Geometry: final body of the model. Coordinates: model frame, mm. A direction names the side the tool comes from. Coordinates: 2 decimals unless noted, no trailing zeros. Loops run counter-clockwise (first coordinate to the right, second up) from the corner with the lowest first, then second, coordinate; pieces in that order, holes last. Notation, with made-up numbers: (-18.75, -11) - (22.25, -11) arc R32 cw to (22.25, 21) - close; hole circle Ø10 at (27, 66.25). An arc over 180 degrees is marked (long way). Answer in a Markdown table with one row per item.
from build123d import *

# Parameters (mm, degrees)
SKETCH1_W           = 101.6
SKETCH1_H           = 101.6
BOSS_EXTRUDE1_DEPTH = 101.6
SKETCH3_W           = 50.8
SKETCH3_H           = 101.6
REVOLVE1_ANGLE      = 90
FILLET1_R           = 2.54


with BuildPart() as part:
    # Sketch1 → Boss-Extrude1 (new body)
    with BuildSketch(Plane(origin=(0, 0, 0), x_dir=(1, 0, 0), z_dir=(0, 1, 0))):
        Rectangle(SKETCH1_W, SKETCH1_H)
    extrude(amount=BOSS_EXTRUDE1_DEPTH)

    # Sketch3 → Revolve1 (revolve)
    with BuildSketch(Plane.XY.offset(50.8)):
        with Locations((25.4, 50.8)):
            Rectangle(SKETCH3_W, SKETCH3_H)
    revolve(axis=Axis((0, 0, 50.8), (0, -1, 0)), revolution_arc=REVOLVE1_ANGLE)

    # Fillet1
    fillet1_edges = [part.edges().sort_by_distance(p)[0] for p in [
        (0, 50.8, 50.8),
    ]]
    fillet(fillet1_edges, radius=FILLET1_R)


solid = part.part
(1) Cut plane B-B on x = -17. Output: boundary loops of the cut face in (y, z).
Verdict:
| item | result |
|---|---|
| outline | (0, -50.8) - (101.6, -50.8) - (101.6, 50.8) - (0, 50.8) - close |
(2) First-contact query: pin 1 Ø5 at (x, y) = (14, 18.5) entering from +Z; pin 2 Ø24 at (x, y) = (-23, 64) entering from +Z; pin 3 Ø14.5 at (y, z) = (71, 66.5) entering from -X. Flat tips, straight axial feed; report the tip coordinate or a pass-through.
Verdict:
| item | result |
|---|---|
| pin 1 | stops at z = 100.28 |
| pin 2 | stops at z = 50.8 |
| pin 3 | stops at x = 0 |
(3) Ray query, probe 1 along Z at (x, y) = (-42, 46.5); probe 2 along X at (y, z) = (5.5, 53); probe 3 along Z at (x, y) = (37.5, 66). Return the intervals inside material, ascending.
Verdict:
| item | result |
|---|---|
| probe 1 | z = -50.8 to 50.8 |
| probe 2 | x = -0.02 to 50.75 |
| probe 3 | z = -50.8 to 85.07 |
(4) Cut plane C-C on z = 65. Output: boundary loops of the cut face in (x, y) (3 decimals), then the cut area to 3 significant figures.
Verdict:
| item | result |
|---|---|
| outline | (0, 0) - (48.775, 0) - (48.775, 101.6) - (0, 101.6) - close |
| area | 4,960 mm² |
(5) Cut plane A-A on y = 23. Output: boundary loops of the cut face in (x, z).
Verdict:
| item | result |
|---|---|
| outline | (-50.8, -50.8) - (50.8, -50.8) - (50.8, 50.8) arc R50.8 ccw to (0, 101.6) - (0, 53.34) arc R2.54 cw to (-2.54, 50.8) - (-50.8, 50.8) - close |
(6) Access query for faces 1 (the face through (0, 52, 77)), 2 (the face through (-50.8, 50, 1)). Directions: +Z, -Z, +X, -X, +Y, -Y. A direction counts if a zero-diameter tool reaches every point of the face in a straight line with its end or side. Return the directions, or none.
Verdict:
| item | result |
|---|---|
| face 1 | +Z, -X, +Y, -Y |
| face 2 | +Z, -Z, -X, +Y, -Y |
